For this review, use the dimensioned drawing (mm, ordinates from the lowest corner) and the shaded views. Coordinates: 2 decimals unless noted, no trailing zeros. Put each result on its own line as item: value.
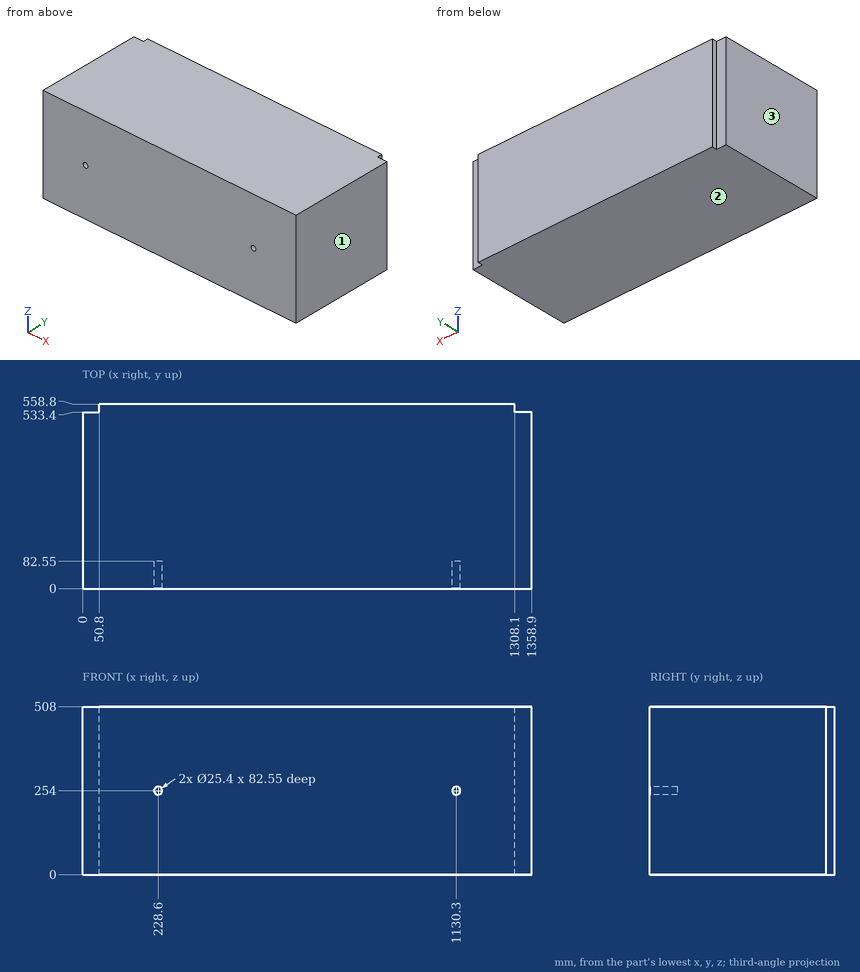
1. To check wall thickness, follow probe 1 along Z at (x, y) = (228.6, 37.5). State the ranges of the line that lie inside material, in increasing order.
Determined:
probe 1: z = 0 to 241.3, 266.7 to 508
2. The part is to be moulded in two halves that separate along X. For the marked faces 1, 2 and 3, say which applies: +X half, -X half, draft (parallel to the pull), parting line (faces both ways), or undercut.
Determined:
face 1: +X half
face 2: draft
face 3: -X half
3. For pin 1 Ø10 at (x, z) = (1132, 107) entering from -Y; pin 2 Ø12.5 at (x, z) = (229, 259) entering from -Y; pin 3 Ø15 at (x, z) = (1330, 342) entering from +Y; pin 4 Ø20.5 at (y, z) = (545, 144) entering from -X, all flat-tipped, find the tip position at first contact; note any pin that passes through.
Determined:
pin 1: stops at y = 0
pin 2: stops at y = 82.55
pin 3: stops at y = 533.4
pin 4: stops at x = 50.8
